Design review of the part built by this model. Coordinates are the model's own, in mm. A direction names the side the tool comes from. Give positions to 0.01 mm unless a question says otherwise; leave off trailing zeros. Loops run counter-clockwise (first coordinate to the right, second up) from the corner with the lowest first, then second, coordinate; pieces in that order, holes last. Notation, with made-up numbers: (46.5, -30.75) -> (61.5, -30.75) arc R25 ccw to (61.5, -9.75) -> close; hole circle Ø5 at (69, 37.25). An arc over 180 degrees is marked (long way). Answer in a Markdown table with one row per item. Add a question column.
(1) Consider section B-B on y = -26.5. Write out the cut boundary in (x, z).
(2) For faces 1 (the flat face through (-19.01, -29.29, 34.51)), 2 (the flat face through (-30, -43, 17)), 3 (the flat face through (-19.01, -29.29, 0.49)), list the 3-axis set-ups (+Z, -Z, +X, -X, +Y, -Y) from which the entire face can be reached by the end or side of a thin tool; tool diameter is ignored.
(3) For line 1 (X direction, y = -10, z = 31.5); line 2 (X direction, y = -21.5, z = 31.5); line 3 (Y direction, x = 0, z = 4.5), list the stretches that pass through material, from the lowest coordinate up.
(4) Consider section A-A on x = 3.5. Write out the cut boundary in (y, z).
(5) Consider section D-D on y = -35.5. Write out the cut boundary in (x, z), then the cut area to 3 significant figures.
(6) For pin 1 (6 mm diameter, centred on x = 1, z = 12, fed in from -Y); pin 2 (1.5 mm diameter, centred on x = -30, z = 18, fed in from -Y); pin 3 (1 mm diameter, centred on x = -8, z = 18, fed in from -Y), all flat-tipped, find the tip position at first contact; note any pin that passes through.
(7) Draft analysis for pull direction X (two halves, no side actions). For faces 4 (the cylindrical face through (-15.115, -13.105, 28.916)), 5 (the flat face through (50, -23, 17)), 6 (the conical face through (-13.22, -10.539, 21.262)), 7 (the flat face through (-1, -13, 0)), state which applies: +X half, -X half, draft (parallel to the pull), parting line (faces both ways), or undercut.
(8) Consider section C-C on z = 3. Write out the cut boundary in (x, y).
from build123d import *

# Parameters (mm, degrees)
BOSS_EXTRUDE1_DEPTH          = 35
CHAMFER1_SIZE                = 1
F_7_0_7_DIAMETER_HOLE1_D     = 7
F_7_0_7_DIAMETER_HOLE1_DEPTH = 12
F_7_0_7_DIAMETER_HOLE1_TIP   = 2.103012167


with BuildPart() as part:
    # Sketch1 → Boss-Extrude1 (new body)
    with BuildSketch(Plane.XY):
        Polygon((50, 0), (-50, 0), (-50, -45), (-30, -45), (-30, -41), (-7, -18), (7, -18), (30, -41), (30, -45), (50, -45), align=None)
    extrude(amount=BOSS_EXTRUDE1_DEPTH)

    # Chamfer1
    chamfer1_edges = [part.edges().sort_by_distance(p)[0] for p in [
        (0, -18, 0),
        (-18.5, -29.5, 0),
        (-30, -43, 0),
        (-40, -45, 0),
        (-50, -22.5, 0),
        (0, 0, 0),
        (50, -22.5, 0),
        (40, -45, 35),
        (40, -45, 0),
        (30, -43, 0),
        (18.5, -29.5, 0),
        (50, -22.5, 35),
        (7, -18, 17.5),
        (-7, -18, 17.5),
        (-30, -41, 17.5),
        (-30, -45, 17.5),
        (-50, -45, 17.5),
        (-50, 0, 17.5),
        (50, 0, 17.5),
        (50, -45, 17.5),
        (30, -45, 17.5),
        (30, -41, 17.5),
        (0, 0, 35),
        (-50, -22.5, 35),
        (-40, -45, 35),
        (-30, -43, 35),
        (-18.5, -29.5, 35),
        (0, -18, 35),
        (18.5, -29.5, 35),
        (30, -43, 35),
    ]]
    chamfer(chamfer1_edges, length=CHAMFER1_SIZE)

    # Ø7.0 (7) Diameter Hole1
    with Locations(Plane.XY.offset(35)):
        with Locations((-13.5, -10), (13.5, -10)):
            Hole(F_7_0_7_DIAMETER_HOLE1_D / 2, depth=F_7_0_7_DIAMETER_HOLE1_DEPTH)
            with Locations((0, 0, -(F_7_0_7_DIAMETER_HOLE1_DEPTH + F_7_0_7_DIAMETER_HOLE1_TIP / 2))):  # 118° drill point
                Cone(0, F_7_0_7_DIAMETER_HOLE1_D / 2, F_7_0_7_DIAMETER_HOLE1_TIP, mode=Mode.SUBTRACT)


solid = part.part
Values follow:
| question | item | result |
|---|---|---|
| 1 | outline | (-50, 1) -> (-49, 0) -> (-16.91, 0) -> (-15.5, 1) -> (-15.5, 34) -> (-16.91, 35) -> (-49, 35) -> (-50, 34) -> close; (15.5, 1) -> (16.91, 0) -> (49, 0) -> (50, 1) -> (50, 34) -> (49, 35) -> (16.91, 35) -> (15.5, 34) -> close |
| 2 | face 1 | +Z, -Y |
| 2 | face 2 | +Z, -Z, -Y |
| 2 | face 3 | -Z, -Y |
| 3 | line 1 | -50 to -17, -10 to 10, 17 to 50 |
| 3 | line 2 | -50 to -10.5, 10.5 to 50 |
| 3 | line 3 | -18 to 0 |
| 4 | outline | (-18, 1) -> (-17, 0) -> (-1, 0) -> (0, 1) -> (0, 34) -> (-1, 35) -> (-17, 35) -> (-18, 34) -> close |
| 5 | outline | (-50, 1) -> (-49, 0) -> (-25.91, 0) -> (-24.5, 1) -> (-24.5, 34) -> (-25.91, 35) -> (-49, 35) -> (-50, 34) -> close; (24.5, 1) -> (25.91, 0) -> (49, 0) -> (50, 1) -> (50, 34) -> (49, 35) -> (25.91, 35) -> (24.5, 34) -> close |
| 5 | area | 1,780 mm2 |
| 6 | pin 1 | y = -18 |
| 6 | pin 2 | y = -44.75 |
| 6 | pin 3 | y = -19.5 |
| 7 | face 4 | undercut |
| 7 | face 5 | +X half |
| 7 | face 6 | undercut |
| 7 | face 7 | draft |
| 8 | outline | (-50, -44) -> (-49, -45) -> (-31, -45) -> (-30, -44) -> (-30, -42) -> (-29.29, -40.29) -> (-7.71, -18.71) -> (-6, -18) -> (6, -18) -> (7.71, -18.71) -> (29.29, -40.29) -> (30, -42) -> (30, -44) -> (31, -45) -> (49, -45) -> (50, -44) -> (50, -1) -> (49, 0) -> (-49, 0) -> (-50, -1) -> close |
